Can you work these out from the drawing? Everything is in mm from the part's minimum corner. Round coordinates to 2 decimals unless told otherwise and drop trailing zeros. Order: outer loops, then holes, each group sorted by start corner. A loop starts at its lowest first (then second) coordinate and runs counter-clockwise, first axis right, second up. Notation, with made-up numbers: (75.5, -11.5) - (97.5, -11.5) arc R16 cw to (97.5, 16.5) - close; hole circle Ø3 at (22.5, -36.75). An arc over 180 degrees is marked (long way). Write item = value, one per line.
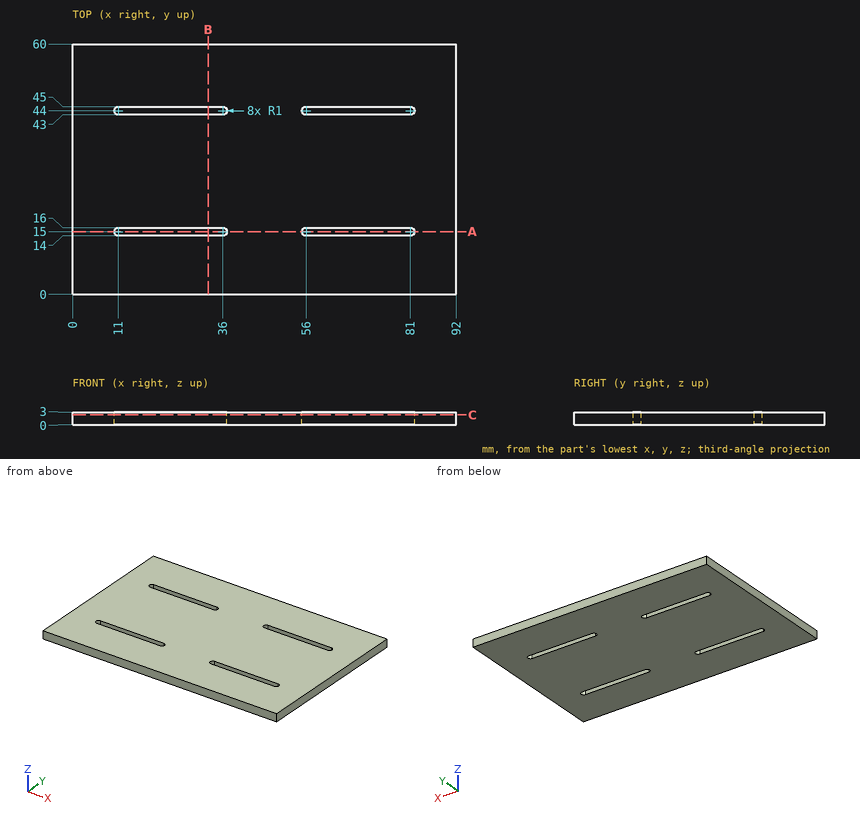
(1) If we section it at C-C (z = 2.4): Write out the boundary of the cut face in (x, y).
Computed:
outline = (0, 0) - (92, 0) - (92, 60) - (0, 60) - close; hole (11, 14) - (36, 14) arc R1 ccw to (36, 16) - (11, 16) arc R1 ccw to start; hole (11, 43) - (36, 43) arc R1 ccw to (36, 45) - (11, 45) arc R1 ccw to start; hole (56, 14) - (81, 14) arc R1 ccw to (81, 16) - (56, 16) arc R1 ccw to start; hole (56, 43) - (81, 43) arc R1 ccw to (81, 45) - (56, 45) arc R1 ccw to start
(2) If I drill on line 1 (Y direction, x = 29, z = 1.4); line 2 (Y direction, x = 10.5, z = 2.75), over which ranges is the centre line in solid material (lowest first)? Write a range as from..to.
Computed:
line_1 = 0..14, 16..43, 45..60
line_2 = 0..14.13, 15.87..43.13, 44.87..60
(3) If we section it at B-B (x = 32.5): Write out the boundary of the cut face in (y, z), plus the area to 3 significant figures.
Computed:
outline = (0, 0) - (14, 0) - (14, 3) - (0, 3) - close; (16, 0) - (43, 0) - (43, 3) - (16, 3) - close; (45, 0) - (60, 0) - (60, 3) - (45, 3) - close
area = 168 mm^2
(4) If we section it at A-A (y = 15): Write out the boundary of the cut face in (x, z).
Computed:
outline = (0, 0) - (10, 0) - (10, 3) - (0, 3) - close; (37, 0) - (55, 0) - (55, 3) - (37, 3) - close; (82, 0) - (92, 0) - (92, 3) - (82, 3) - close
